Geometry: final body of the model. Coordinates: model frame, mm. A direction names the side the tool comes from. Coordinates: 2 decimals unless noted, no trailing zeros. Write each loop counter-clockwise with the first axis right and the second up, starting at its lowest first coordinate (ties: lowest second). Pieces come first, ordered by that corner, then holes. Notation, with made-up numbers: M -39,-25.75 L -33,-25.75 A28 cw -33,0.25 Z; hole C -37.5,12 d10. An arc over 180 degrees is marked long. Write item = value, one per line. Start each with the question number.
Item 1: Pull-direction query (X, two-part tool) for faces 1 (the cylindrical face through (-66.307, 34.019, 1.602)), 2 (the flat face through (-30, 41.309, 2)), 3 (the flat face through (-22, 47.809, 2)); classes: +X half, -X half, draft (parallel to the pull), parting line (faces both ways), or undercut.
Item 2: Section A-A on x = -30. Output: boundary loops of the cut face in (y, z), plus the area to 4 significant figures.
Item 3: Ray query, L1, parallel to Y at x = -29, z = 2; L2, parallel to X at y = 30.5, z = 1.2; L3, parallel to X at y = 29.25, z = 3. Return the intervals inside material, ascending. Write a range as [from, to].
Item 4: First-contact query: pin 1 Ø1.5 at (y, z) = (26.5, 1.5) entering from +X. Flat tip, straight axial feed; report the tip coordinate or a pass-through.
Item 5: Reachability of faces 4 (the flat face through (-22, 34, 0)), 5 (the flat face through (-30, 27.309, 2)) from +Z, -Z, +X, -X, +Y, -Y: full face, straight path, thin tool, end or side. Return the list, or none.
Item 6: Section D-D on x = -58. Output: boundary loops of the cut face in (y, z).
Item 7: Section C-C on z = 1.1. Output: boundary loops of the cut face in (x, y).
Autodesk Inventor part; units mm, degrees
ref_plane "YZ Plane" through (0, 0, 0) normal (1, 0, 0) x (0, 1, 0)
ref_plane "XZ Plane" through (0, 0, 0) normal (0, 1, 0) x (-1, 0, 0)
ref_plane "XY Plane" through (0, 0, 0) normal (0, 0, 1) x (1, 0, 0)
sketch "Block1" plane through (0, 0, 0) normal (0, 0, 1) x (1, 0, 0)
  circle A0 centre (74.029, 24.2723) radius 1
  line L0 (49.279, 30.4723) -> (71.779, 30.4723)
  line L1 (71.779, 30.4723) -> (71.779, 18.0723)
  line L2 (71.779, 18.0723) -> (49.279, 18.0723)
  line L3 (49.279, 18.0723) -> (49.279, 30.4723)
  line L4 (49.279, 30.4723) -> (44.779, 30.4723)
  line L5 (44.779, 30.4723) -> (44.779, 18.0723)
  line L6 (44.779, 18.0723) -> (49.279, 18.0723)
  line L7 (49.279, 18.0723) -> (49.279, 30.4723)
  line L8 (71.779, 30.4723) -> (76.279, 30.4723)
  line L9 (76.279, 30.4723) -> (76.279, 18.0723)
  line L10 (76.279, 18.0723) -> (71.779, 18.0723)
  line L11 (71.779, 18.0723) -> (71.779, 30.4723)
  line L12 (44.779, 24.2723) -> (76.279, 24.2723) construction
  line L13 (47.029, 30.4723) -> (47.029, 18.0723) construction
  circle A1 centre (47.029, 24.2723) radius 1
  line L14 (74.029, 30.4723) -> (74.029, 18.0723) construction
  point P0 (60.979, 24.0984)
  dimension "d7" = 22.5
  dimension "d8" = 12.4
  dimension "d9" = 4.5
  dimension "d10" = 4.5
  dimension "d11" = 2
  dimension "d12" = 2
sketch "Sketch1" plane through (0, 0, 0) normal (0, 0, 1) x (1, 0, 0)
  line L0 (-92.7646, -8.503) -> (-89.7646, -8.503)
  line L1 (-89.7646, -8.503) -> (-89.7646, -11.753)
  line L2 (-89.7646, -11.753) -> (-92.7646, -11.753)
  line L3 (-92.7646, -11.753) -> (-92.7646, -8.503)
  line L4 (-92.7646, -21.6527) -> (-89.7646, -21.6527)
  line L5 (-89.7646, -21.6527) -> (-89.7646, -21.7527)
  line L6 (-89.7646, -21.7527) -> (-92.7646, -21.7527)
  line L7 (-92.7646, -21.7527) -> (-92.7646, -21.6527)
  line L8 (-66.3097, 47.8088) -> (23.6903, 47.8088)
  line L9 (23.6903, 47.8088) -> (23.6903, 20.8088)
  line L10 (23.6903, 20.8088) -> (-66.3097, 20.8088)
  line L11 (-66.3097, 20.8088) -> (-66.3097, 47.8088)
  line L12 (-66.3097, 34.3088) -> (23.6903, 34.3088) construction
  line L13 (-31.3097, 41.3088) -> (-28.0597, 41.3088)
  line L14 (-28.0597, 41.3088) -> (-28.0597, 27.3088)
  line L15 (-28.0597, 27.3088) -> (-31.3097, 27.3088)
  line L16 (-31.3097, 27.3088) -> (-31.3097, 41.3088)
  line L17 (-31.3097, 34.3088) -> (-28.0597, 34.3088) construction
  line L18 (-53.3097, 47.8088) -> (-53.3097, 20.8088) construction
  line L19 (-21.3097, 47.8088) -> (-21.3097, 20.8088) construction
  line L20 (10.6903, 47.8088) -> (10.6903, 20.8088) construction
  arc A0 (-53.3097, 47.8088) -> (-53.3097, 20.8088) centre (-52.8001, 34.3088) ccw
  arc A1 (10.6903, 20.8088) -> (10.6903, 47.8088) centre (10.1806, 34.3088) ccw
  point P0 (0, 0)
  dimension "d0" = 3
  dimension "mat" = 3.25
  dimension "d2" = 3
  dimension "d3" = 0.1
  dimension "d23" = 90
  dimension "d24" = 27
  dimension "d29" = 3.25
  dimension "d30" = 14
  dimension "d31" = 35
  dimension "d36" = 13
  dimension "d38" = 13
extrude "Extrusion5" add sketch "Sketch1" along normal blind 3.25 contours L8 A1 L10 A0
equation "\"d29\" = mat"
equation "\"d42\" = mat"
properties part number "arm-servo"
Responses:
q1.face_1 = -X half
q1.face_2 = undercut
q1.face_3 = draft
q2.outline = M 20.81,0 L 27.31,0 L 27.31,3.25 L 20.81,3.25 Z; M 41.31,0 L 47.81,0 L 47.81,3.25 L 41.31,3.25 Z
q2.area = 42.25 mm²
q3.L1 = [20.81, 27.31], [41.31, 47.81]
q3.L2 = [-65.76, -31.31], [-28.06, 23.14]
q3.L3 = [-65.33, -31.31], [-28.06, 22.71]
q4.pin_1 = 21.7
q5.face_4 = -Z, +X, -X, +Y, -Y
q5.face_5 = +Z, -Z
q6.outline = M 21.84,0 L 46.78,0 L 46.78,3.25 L 21.84,3.25 Z
q7.outline = M -53.31,20.81 L 10.69,20.81 A13.51 ccw 10.69,47.81 L -53.31,47.81 A13.51 ccw Z; hole M -31.31,27.31 L -28.06,27.31 L -28.06,41.31 L -31.31,41.31 Z
